Model file for the job. Use its own axes, mm. A direction names the side the tool comes from. Give positions to 0.01 mm unless a question says otherwise; leave off trailing zeros. Write each loop counter-clockwise with the first axis right and the second up, starting at its lowest first coordinate (ties: lowest second). Pieces come first, ordered by that corner, then holes. Notation, with made-up numbers: (-39.5, 53) - (-21.5, 53) arc R22 cw to (-21.5, 60) - close; hole circle Ø5 at (-34.75, 4.25). An arc over 180 degrees is marked (long way). Use CSV: the item, a comma, the result in double quotes.
from build123d import *

# Parameters (mm, degrees)
SKETCH_1_W             = 495
SKETCH_1_H             = 60
EXTRUDE_1_DEPTH        = 3
SKETCH_2_W             = 3
SKETCH_2_H             = 60
EXTRUDE_2_DEPTH        = 200
EXTRUDE_3_DEPTH        = 60
SKETCH_4_R             = 10
EXTRUDE_4_DEPTH        = 25
SKETCH_5_R             = 5.5
CUT_EXTRUDE_1_DEPTH    = 529.441103625
PATTERN_LINEAR_1_COUNT = 8
PATTERN_LINEAR_1_PITCH = 60
FILLET_1_R             = 30
SKETCH_6_W             = 203
SKETCH_6_H             = 5
EXTRUDE_5_DEPTH        = 5
SKETCH_7_W             = 203
SKETCH_7_H             = 5
EXTRUDE_6_DEPTH        = 5
FILLET_2_R             = 5
FILLET_3_R             = 5


with BuildPart() as part:
    # 草图1 → 凸台-拉伸1 (new body)
    with BuildSketch(Plane.XY):
        with Locations((247.5, 30)):
            Rectangle(SKETCH_1_W, SKETCH_1_H)
    extrude(amount=EXTRUDE_1_DEPTH)

    # 草图2 → 凸台-拉伸2 (add)
    with BuildSketch(Plane(origin=(0, 0, 0), x_dir=(-1, 0, 0), z_dir=(0, 0, -1))):
        with Locations((-493.5, 30)):
            Rectangle(SKETCH_2_W, SKETCH_2_H)
        with Locations((-1.5, 30)):
            Rectangle(SKETCH_2_W, SKETCH_2_H)
    extrude(amount=EXTRUDE_2_DEPTH)

    # 草图3 → 凸台-拉伸3 (add)
    with BuildSketch(Plane.XZ):
        Polygon((3, -20), (23, 0), (3, 0), align=None)
        Polygon((472, 0), (492, 0), (492, -20), align=None)
    extrude(amount=-EXTRUDE_3_DEPTH)

    # 草图4 → 凸台-拉伸4 (add)
    with BuildSketch(Plane(origin=(0, 0, 0), x_dir=(-1, 0, 0), z_dir=(0, 0, -1))):
        with Locations((-457.5, 30)):
            Circle(SKETCH_4_R)
    extrude_4 = extrude(amount=EXTRUDE_4_DEPTH)

    # 草图5 → 切除-拉伸1 (cut, through all)
    with BuildSketch(Plane(origin=(0, 0, -25), x_dir=(-1, 0, 0), z_dir=(0, 0, -1))):
        with Locations((-457.5, 30)):
            Circle(SKETCH_5_R)
    cut_extrude_1 = extrude(amount=-CUT_EXTRUDE_1_DEPTH, mode=Mode.SUBTRACT)

    # 阵列(线性)1: 凸台-拉伸4, 切除-拉伸1 ×8
    with Locations(*[(-i * PATTERN_LINEAR_1_PITCH, 0, 0) for i in range(1, PATTERN_LINEAR_1_COUNT)]):
        add(extrude_4)
        add(cut_extrude_1, mode=Mode.SUBTRACT)

    # 圆角1
    fillet_1_edges = [part.edges().sort_by_distance(p)[0] for p in [
        (3, 30, -20),
        (492, 30, -20),
    ]]
    fillet(fillet_1_edges, radius=FILLET_1_R)

    # 草图6 → 凸台-拉伸5 (add)
    with BuildSketch(Plane.ZY):
        with Locations((-98.5, 2.5)):
            Rectangle(SKETCH_6_W, SKETCH_6_H)
    extrude(amount=EXTRUDE_5_DEPTH)

    # 草图7 → 凸台-拉伸6 (add)
    with BuildSketch(Plane(origin=(495, 0, 0), x_dir=(0, 0, -1), z_dir=(1, 0, 0))):
        with Locations((98.5, 2.5)):
            Rectangle(SKETCH_7_W, SKETCH_7_H)
    extrude(amount=EXTRUDE_6_DEPTH)

    # 圆角2
    fillet_2_edges = [part.edges().sort_by_distance(p)[0] for p in [
        (0, 5, -98.5),
    ]]
    fillet(fillet_2_edges, radius=FILLET_2_R - 0.0001)  # a hair under: the kernel refuses the full size

    # 圆角3
    fillet_3_edges = [part.edges().sort_by_distance(p)[0] for p in [
        (495, 5, -98.5),
    ]]
    fillet(fillet_3_edges, radius=FILLET_3_R - 0.0001)  # a hair under: the kernel refuses the full size


solid = part.part
(1) Flat gauge pins, fed straight in: P1, Ø5, axis at x = 54.5, y = 20, coming from the -Z side; P2, Ø10, axis at x = 400.5, y = 27, coming from the -Z side; P3, Ø6.5, axis at x = 97.5, y = 30, coming from the +Z side; P4, Ø4, axis at y = 33.5, z = -68.5, coming from the +X side. Where does each tip first touch, or does it go through?
Checked values:
P1,"stops at z = 0"
P2,"stops at z = -25"
P3,"passes through"
P4,"stops at x = 495"
(2) Wall check: probe 1 along X at (y, z) = (3, -134); probe 2 along Y at (x, z) = (397.5, -16); probe 3 along X at (y, z) = (34.5, -161). Give the ranges that are in metal, low to high. Write a range as [from, to].
Checked values:
probe 1,"x = [-5, 3], [492, 500]"
probe 2,"y = [20, 24.5], [35.5, 40]"
probe 3,"x = [0, 3], [492, 495]"
(3) Saw through at B-B, the plane x = 217.5. List the corners of the cut face in (y, z).
Checked values:
outline,"(0, 0) - (20, 0) - (20, -25) - (24.5, -25) - (24.5, 3) - (0, 3) - close; (35.5, -25) - (40, -25) - (40, 0) - (60, 0) - (60, 3) - (35.5, 3) - close"
(4) Saw through at C-C, the plane y = 30. Count the separate pieces of the cut face and the enclosed holes in it, then the cut area to 3 significant figures.
Checked values:
separate pieces,"9"
enclosed holes,"0"
area,"4,660 mm^2"
(5) 3-axis set-ups, long thin cutter, end or side, ignore diameter. For faces 1 (the face through (393, 26, -25)), 2 (the face through (207.96, 33, -12.32)), 3 (the face through (0, 35, -100)), 4 (the face through (332.254, 31.652, -11.196)), 5 (the face through (244, 30, 3)): which of +Z, -Z, +X, -X, +Y, -Y reach the whole face in a straight line?
Checked values:
face 1,"-Z, +Y, -Y"
face 2,"-Z"
face 3,"+Z, -Z, -X, +Y"
face 4,"+Z, -Z"
face 5,"+Z, +X, -X, +Y, -Y"
(6) Pull direction Y, two halves, no side cores. Call faces 6 (the face through (452.254, 31.652, -11.196)), 7 (the face through (495, 35, -97)), 8 (the face through (447.96, 33, -12.32)): released by +Y, released by -Y, zero draft, split by the parting line, or undercut.
Checked values:
face 6,"undercut"
face 7,"zero draft"
face 8,"split by the parting line"
